The listing builds one solid part. Answer for the finished solid, in the listing's coordinates (mm). Round coordinates to 2 decimals unless told otherwise and drop trailing zeros. Order: outer loops, then holes, each group sorted by start corner. A loop starts at its lowest first (then second) coordinate and runs counter-clockwise, first axis right, second up. Notation, with made-up numbers: (-19.75, 9.25) -> (-6.75, 9.25) arc R23 ccw to (-6.75, 45.25) -> close; hole circle Ø3 at (22, 87). An arc over 180 degrees is marked (long way). Return JSON: item names as keys, results as strings. Group by question number.
(1) Consider line 1 (X direction, y = -3, z = -24); line 2 (Y direction, x = -4, z = 0.5); line 3 (Y direction, x = 4.5, z = -6). Determine where each line is inside the solid, lowest interval first. Write a range as [from, to].
(2) Each of these flat-tipped pins is pushed along its axis until it touches: pin 1 (4 mm diameter, centred on y = -1, z = -2, fed in from +X); pin 2 (3 mm diameter, centred on x = -4.5, y = -2.5, fed in from +Z); pin 3 (1 mm diameter, centred on x = -1.5, y = -6, fed in from +Z). Where does it stop, or does it pass through?
(3) The part is cut by section A-A (z = -25.5). Determine the outline of the cut face in (x, y).
from build123d import *

# Parameters (mm, degrees)
F1_DEPTH = 7.112
F2_R     = 3.0734


with BuildPart() as f1:
    # F0 (on Front) → F1 (new body)
    with BuildSketch(Plane.XZ):
        with BuildLine():
            Line((-5.833062, 5.073665), (-5.833062, -2.089096))
            ThreePointArc((-5.833062, -2.089096), (-0.414611, 3.329354), (5.003839, -2.089096))
            Line((5.003839, -2.089096), (5.003839, 1.10841))
            Line((5.003839, 1.10841), (5.003839, 9.281913))
            ThreePointArc((5.003839, 9.281913), (-0.414611, 14.700363), (-5.833062, 9.281913))
            Line((-5.833062, 9.281913), (-5.833062, 5.073665))
        make_face()
        with BuildLine():
            Line((5.003839, -2.089096), (-5.833062, -2.089096))
            ThreePointArc((-5.833062, -2.089096), (-0.414611, -7.507547), (5.003839, -2.089096))
        make_face()
        with BuildLine():
            ThreePointArc((5.003839, -2.089096), (-0.414611, 3.329354), (-5.833062, -2.089096))
            Line((-5.833062, -2.089096), (5.003839, -2.089096))
        make_face()
        with BuildLine():
            Line((-5.833062, -2.089096), (-5.833062, -27.969601))
            ThreePointArc((-5.833062, -27.969601), (-0.414611, -33.388051), (5.003839, -27.969601))
            Line((5.003839, -27.969601), (5.003839, -9.071903))
            Line((5.003839, -9.071903), (5.003839, -2.089096))
            ThreePointArc((5.003839, -2.089096), (-0.414611, -7.507547), (-5.833062, -2.089096))
        make_face()
    extrude(amount=F1_DEPTH)

    # F2
    f2_edges = [f1.edges().sort_by_distance(p)[0] for p in [
        (5.003839, -7.112, -9.343844),
        (5.003839, 0, -9.343844),
        (-0.414611, -7.112, 14.700363),
        (-0.414611, 0, 14.700363),
        (-0.414611, 0, -33.388051),
        (-0.414611, -7.112, -33.388051),
        (-5.833062, 0, -9.343844),
        (-5.833062, -7.112, -9.343844),
    ]]
    fillet(f2_edges, radius=F2_R)


solid = f1.part
Answer below:
{
 "1": {"line 1": "x = [-5.83, 5]", "line 2": "y = [-6.85, -0.26]", "line 3": "y = [-5.72, -1.39]"},
 "2": {"pin 1": "stops at x = 5", "pin 2": "stops at z = 14.01", "pin 3": "stops at z = 14.23"},
 "3": {"outline": "(-5.83, -4.04) arc R3.07 ccw to (-2.76, -7.11) -> (1.93, -7.11) arc R3.07 ccw to (5, -4.04) -> (5, -3.07) arc R3.07 ccw to (1.93, 0) -> (-2.76, 0) arc R3.07 ccw to (-5.83, -3.07) -> close"}
}
